Geometry check sheet. Reference: the model listing, model coordinates, mm. A direction names the side the tool comes from. Round coordinates to 2 decimals unless told otherwise and drop trailing zeros. Loops run counter-clockwise (first coordinate to the right, second up) from the corner with the lowest first, then second, coordinate; pieces in that order, holes last. Notation, with made-up numbers: M -14,63 L 44,63 A10 cw 44,76 Z; hole C 57.5,34 d10. An arc over 180 degrees is marked long. Write item = value, one per line.
from build123d import *

# Parameters (mm, degrees)
PAD_DEPTH    = 8.89
PAD001_DEPTH = 1.524


with BuildPart() as part:
    # Sketch → Pad (new body)
    with BuildSketch(Plane.XY):
        with BuildLine():
            Line((0, 0), (34.67, 0))
            Line((34.67, 0), (34.67, 4))
            Line((32.878183, 12.345886), (34.67, 4))
            Line((32.584282, 12.256473), (32.878183, 12.345886))
            Line((30.236841, 10.317895), (32.584282, 12.256473))
            Line((31.895653, 10.315125), (30.236841, 10.317895))
            Line((33.146309, 4.011625), (31.895653, 10.315125))
            Line((17.790159, 3.913346), (33.146309, 4.011625))
            Line((18.678085, 10.301132), (17.790159, 3.913346))
            Line((20.137171, 10.305716), (18.678085, 10.301132))
            Line((17.736418, 12.384692), (20.137171, 10.305716))
            Line((17.467266, 12.41508), (17.736418, 12.384692))
            Line((16.074211, 3.934741), (17.467266, 12.41508))
            Line((14.35, 3.937935), (16.074211, 3.934741))
            Line((14.35, 15), (14.35, 3.937935))
            Line((0, 15), (14.35, 15))
            Line((0, 11), (0, 15))
            Line((3.540018, 11), (0, 11))
            ThreePointArc((6.35, 4), (10.121472, 9.577967), (3.540018, 11))
            Line((0, 4), (6.35, 4))
            Line((0, 0), (0, 4))
        make_face()
    extrude(amount=PAD_DEPTH)

    # Sketch001 → Pad001 (new body)
    with BuildSketch(Plane.XY.offset(8.89)):
        Polygon((16.09544, 3.889412), (17.92443, 5.005656), (33.057573, 5.005656), (34.640282, 3.938822), align=None)
    extrude(amount=-PAD001_DEPTH)


solid = part.part
(1) Release check for a two-part mould opening along X. For faces 1 (the flat face through (25.6, 4.5, 7.366)), 2 (the flat face through (25, 5.006, 8)), 3 (the flat face through (17, 0, 4)), 4 (the flat face through (0, 2, 4)) record: released by +X, released by -X, zero draft, split by the parting line, or undercut.
Result set:
face_1 = undercut
face_2 = undercut
face_3 = zero draft
face_4 = released by -X
(2) Material ranges on line 1 along Y through (x, z) = (6.35, 4.25); line 2 along X through (y, z) = (8.5, 1.5); line 3 along Y through (x, z) = (14.5, 3), recorded low to high. Write a range as from..to.
Result set:
line_1 = 0..4, 12.13..15
line_2 = 10.39..14.35, 16.82..18.43, 32.26..33.7
line_3 = 0..3.94
(3) Depth check by flat-ended pin: pin 1 Ø8 at (x, y) = (20, 9) entering from -Z; pin 2 Ø0.5 at (x, y) = (29, 4.5) entering from -Z; pin 3 Ø2.5 at (y, z) = (9, 6) entering from +X; pin 4 Ø1.7 at (x, z) = (25.5, 8) entering from +Y. Enter the tip coordinate at first touch or a pass-through.
Result set:
pin_1 = 0
pin_2 = 7.37
pin_3 = 33.86
pin_4 = 5.01
(4) Sectioned sample at D-D on x = 4. Record the cut outline in (y, z), then the cut area to 3 significant figures.
Result set:
outline = M 0,0 L 4,0 L 4,8.89 L 0,8.89 Z; M 11.38,0 L 15,0 L 15,8.89 L 11.38,8.89 Z
area = 67.7 mm2
(5) Tool access check on faces 5 (the flat face through (17, 6, 0)), 6 (the flat face through (18.92, 11.36, 4.38)), 7 (the flat face through (2, 11, 4)). Record the directions out of +Z, -Z, +X, -X, +Y, -Y that give a thin tool (end or side, any length) a straight path to the whole face; none if there is none.
Result set:
face_5 = -Z, +X, -X, +Y, -Y
face_6 = +Z, -Z, +Y
face_7 = +Z, -Z, -X
(6) Sectioned sample at B-B on y = 9.5. Record the cut outline in (x, z).
Result set:
outline = M 10.15,0 L 14.35,0 L 14.35,8.89 L 10.15,8.89 Z; M 16.99,0 L 18.57,0 L 18.57,8.89 L 16.99,8.89 Z; M 32.06,0 L 33.49,0 L 33.49,8.89 L 32.06,8.89 Z
(7) Sectioned sample at C-C on x = 31. Record the cut outline in (y, z), then the cut area to 3 significant figures.
Result set:
outline = M 0,0 L 4,0 L 4,7.37 L 5.01,7.37 L 5.01,8.89 L 0,8.89 Z; M 10.32,0 L 10.95,0 L 10.95,8.89 L 10.32,8.89 Z
area = 42.7 mm2
(8) Sectioned sample at A-A on z = 8.25. Record the cut outline in (x, y), then the cut area to 3 significant figures.
Result set:
outline = M 0,0 L 34.67,0 L 34.67,4 L 32.88,12.35 L 32.58,12.26 L 30.24,10.32 L 31.9,10.32 L 32.95,5.01 L 17.94,5.01 L 18.68,10.3 L 20.14,10.31 L 17.74,12.38 L 17.47,12.42 L 16.07,3.93 L 14.35,3.94 L 14.35,15 L 0,15 L 0,11 L 3.54,11 A4.06 cw long 6.35,4 L 0,4 Z
area = 265 mm2
